```python
from build123d import *

# Parameters (mm, degrees)
SKETCH1_W           = 100
SKETCH1_H           = 50
BOSS_EXTRUDE1_DEPTH = 20
SKETCH2_R           = 12.5
SKETCH2_W           = 20
SKETCH2_H           = 20
BOSS_EXTRUDE2_DEPTH = 10


with BuildPart() as part:
    # Sketch1 → Boss-Extrude1 (new body)
    with BuildSketch(Plane.XY):
        with Locations((50, 25)):
            Rectangle(SKETCH1_W, SKETCH1_H)
    extrude(amount=BOSS_EXTRUDE1_DEPTH)

    # Sketch2 → Boss-Extrude2 (add)
    with BuildSketch(Plane.XY.offset(20)):
        with Locations((72.515853305, 25.964965142)):
            Circle(SKETCH2_R)
        with Locations((26.226220042, 25.028693536)):
            Rectangle(SKETCH2_W, SKETCH2_H)
    extrude(amount=BOSS_EXTRUDE2_DEPTH)


solid = part.part
```
Verification items for the finished model (mm, model axes). A direction names the side the tool comes from. Round coordinates to 2 decimals unless told otherwise and drop trailing zeros. Write each loop counter-clockwise with the first axis right and the second up, starting at its lowest first coordinate (ties: lowest second). Pieces come first, ordered by that corner, then holes. Notation, with made-up numbers: (74.5, 64) - (107.5, 64) arc R27 cw to (107.5, 85) - close; hole circle Ø8 at (-2.5, 47). An arc over 180 degrees is marked (long way). Answer as a JSON object with one key per item and string values. Group by question number.
Q1. Mould release check, pull along X, two halves, no side actions. Record for faces 4 (the flat face through (16.226, 25, 25)), 5 (the flat face through (49, 0, 10)), 6 (the flat face through (100, 25, 10)), 7 (the cylindrical face through (62.596, 18.359, 24.93)): released by +X, released by -X, zero draft, split by the parting line, or undercut.
Q2. Thickness scan on line 1 (Z direction, x = 96.5, y = 37.5); line 2 (X direction, y = 15.5, z = 24.25); line 3 (Y direction, x = 25, z = 25.75). Record the ranges inside material, lowest first.
Q3. Go/stop test with flat-tipped pins: pin 1 Ø3 at (x, z) = (22, 25.5) entering from -Y; pin 2 Ø3 at (y, z) = (20, 25.5) entering from +X; pin 3 Ø10 at (x, y) = (47, 9.5) entering from +Z. Record where each tip stops, or that it passes through.
Q4. Tool access check on faces 1 (the flat face through (26, 35.029, 25)), 2 (the flat face through (36.226, 25, 25)), 3 (the flat face through (26, 15.029, 25)). Record the directions out of +Z, -Z, +X, -X, +Y, -Y that give a thin tool (end or side, any length) a straight path to the whole face; none if there is none.
Q5. Section check A-A, the plane x = 21. Enter the section's corners in (y, z).
Q6. Section check C-C, the plane y = 27.5. Enter the section's corners in (x, z).
Q7. Section check D-D, the plane y = 18. Enter the section's corners in (x, z).
Q8. Section check B-B, the plane z = 23.25. Enter the section's corners in (x, y).
Found:
{
 "1": {"face 4": "released by -X", "face 5": "zero draft", "face 6": "released by +X", "face 7": "undercut"},
 "2": {"line 1": "z = 0 to 20", "line 2": "x = 16.23 to 36.23, 65.68 to 79.35", "line 3": "y = 15.03 to 35.03"},
 "3": {"pin 1": "stops at y = 15.03", "pin 2": "stops at x = 84.19", "pin 3": "stops at z = 20"},
 "4": {"face 1": "+Z, -X, +Y", "face 2": "+Z, +Y, -Y", "face 3": "+Z, -X, -Y"},
 "5": {"outline": "(0, 0) - (50, 0) - (50, 20) - (35.03, 20) - (35.03, 30) - (15.03, 30) - (15.03, 20) - (0, 20) - close"},
 "6": {"outline": "(0, 0) - (100, 0) - (100, 20) - (84.92, 20) - (84.92, 30) - (60.11, 30) - (60.11, 20) - (36.23, 20) - (36.23, 30) - (16.23, 30) - (16.23, 20) - (0, 20) - close"},
 "7": {"outline": "(0, 0) - (100, 0) - (100, 20) - (82.15, 20) - (82.15, 30) - (62.88, 30) - (62.88, 20) - (36.23, 20) - (36.23, 30) - (16.23, 30) - (16.23, 20) - (0, 20) - close"},
 "8": {"outline": "(16.23, 15.03) - (36.23, 15.03) - (36.23, 35.03) - (16.23, 35.03) - close; circle Ø25 at (72.52, 25.96)"}
}
